from build123d import *

# Parameters (mm, degrees)
EXTRUDE_1_DEPTH = 169


with BuildPart() as part:
    # 草图1 → 凸台-拉伸1 (new body)
    with BuildSketch(Plane.XY):
        with BuildLine():
            Line((0, 0), (142, 0))
            Line((142, 0), (142, 23))
            ThreePointArc((142, 23), (139.071067812, 30.071067812), (132, 33))
            Line((132, 33), (10, 33))
            ThreePointArc((10, 33), (2.928932188, 30.071067812), (0, 23))
            Line((0, 23), (0, 0))
        make_face()
    extrude(amount=EXTRUDE_1_DEPTH)


solid = part.part
Model file for the job. Use its own axes, mm. Give positions to 0.01 mm unless a question says otherwise; leave off trailing zeros. Loops run counter-clockwise (first coordinate to the right, second up) from the corner with the lowest first, then second, coordinate; pieces in that order, holes last.
Item 1: Slice it at A-A (y = 28). Write the cut outline in (x, z), plus the area to 3 significant figures.
Check values:
outline: (1.34, 0) - (140.66, 0) - (140.66, 169) - (1.34, 169) - close
area: 23,500 mm2
Item 2: Drop a flat-ended pin along its axis: P1, Ø4, axis at x = 78.5, z = 31, coming from the -Y side. Give the stop position or say it passes through.
Check values:
P1: stops at y = 0
Item 3: Drill centre lines: line 1 along X through (y, z) = (30.5, 109); line 2 along X through (y, z) = (28.5, 124); line 3 along Y through (x, z) = (136, 108.5). Where is each one in solid material? Low to high.
Check values:
line 1: x = 3.39 to 138.61
line 2: x = 1.65 to 140.35
line 3: y = 0 to 32.17
